Can you work these out from the model? Positions are in its coordinate system, mm. A direction names the side the tool comes from. Coordinates: 2 decimals unless noted, no trailing zeros. Write each loop counter-clockwise with the first axis right and the second up, starting at its lowest first coordinate (ties: lowest second). Pieces come first, ordered by that corner, then holes.
Autodesk Inventor part; units mm, degrees
ref_plane "YZ Plane" through (0, 0, 0) normal (1, 0, 0) x (0, 1, 0)
ref_plane "XZ Plane" through (0, 0, 0) normal (0, 1, 0) x (-1, 0, 0)
ref_plane "XY Plane" through (0, 0, 0) normal (0, 0, 1) x (1, 0, 0)
sketch "Sketch1" plane through (0, 0, 0) normal (0, 0, 1) x (1, 0, 0)
  point P0 (0, 0)
sketch "Sketch2" plane through (0, 0, 0) normal (0, 0, 1) x (1, 0, 0)
  line L0 (0, 0) -> (-34, 0)
  line L1 (-34, 0) -> (-34, 15)
  line L2 (-34, 15) -> (0, 15)
  line L3 (0, 15) -> (0, 0)
  dimension "d0" = 34
  dimension "d1" = 15
extrude "Extrusion1" add sketch "Sketch2" along normal blind 1
sketch "Sketch3" plane through (0, 0, 1) normal (0, 0, 1) x (1, 0, 0)
  line L0 (0, 0) -> (0, 15)
  point P0 (-8, 7.5)
  point P1 (-22, 7.5)
  dimension "d4" = 14
  dimension "d5" = 8
hole "Hole1" at (-22, 7.5, 1) at (-8, 7.5, 1) direction (0, 0, -1) diameter 4.5 end through all
sketch "Sketch4" plane through (0, 0, 1) normal (0, 0, 1) x (1, 0, 0)
  line L0 (-24, 15) -> (-6, 15)
  line L1 (-6, 15) -> (-6, 3)
  line L2 (-6, 3) -> (-24, 3)
  line L3 (-24, 3) -> (-24, 15)
  line L4 (0, 0) -> (0, 15)
  dimension "d13" = 18
  dimension "d14" = 12
  dimension "d15" = 6
extrude "Extrusion2" add sketch "Sketch4" along normal blind 2.8
sketch "Sketch6" plane through (0, 0, 3.8) normal (0, 0, 1) x (1, 0, 0)
  arc A0 (-24, 6.4692) -> (-24, 8.5308) centre (-22, 7.5) ccw
  arc A1 (-6, 8.5308) -> (-6, 6.4692) centre (-8, 7.5) ccw
  point P0 (0, 0)
hole "Hole2" at (-8, 7.5, 3.8) at (-22, 7.5, 3.8) direction (0, 0, -1) diameter 2 end through all
sketch "Sketch5" plane through (0, 0, 3.8) normal (0, 0, 1) x (1, 0, 0)
  line L0 (-34, 15) -> (0, 15)
  line L1 (-18.5, 15) -> (-11.5, 15)
  line L2 (-11.5, 15) -> (-11.5, 3)
  line L3 (-11.5, 3) -> (-18.5, 3)
  line L4 (-18.5, 3) -> (-18.5, 15)
  line L5 (-24, 15) -> (-24, 3)
  line L6 (-6, 3) -> (-6, 15)
  point P0 (0, 0)
  dimension "d18" = 7
  dimension "d19" = 0
  dimension "d20" = 5.5
  dimension "d21" = 5.5
extrude "Extrusion3" add sketch "Sketch5" along normal blind 5.8
sketch "Sketch7" plane through (-34, 15, 0) normal (0, 1, 0) x (1, 0, 0)
  line L0 (0, 0) -> (34, 0)
  line L1 (0, 0) -> (0, -1)
  line L2 (10, -1) -> (0, -1)
  line L3 (10, -1) -> (10, -3.8)
  line L4 (15.5, -3.8) -> (10, -3.8)
  line L5 (15.5, -3.8) -> (15.5, -9.6)
  line L6 (22.5, -9.6) -> (15.5, -9.6)
  line L7 (22.5, -3.8) -> (22.5, -9.6)
  line L8 (28, -3.8) -> (22.5, -3.8)
  line L9 (28, -1) -> (28, -3.8)
  line L10 (34, -1) -> (28, -1)
  line L11 (34, 0) -> (34, -1)
  line L12 (15.5, -3.8) -> (15.5, -9.6)
  line L13 (22.5, -8.35) -> (15.5, -8.35)
  line L14 (15.5, -8.35) -> (15.5, -5)
  line L15 (15.5, -5) -> (22.5, -5)
  line L16 (22.5, -5) -> (22.5, -8.35)
  dimension "d31" = 5
  dimension "d32" = 1.25
extrude "Extrusion4" cut sketch "Sketch7" against normal blind 6 contours L15 L7 L13 L5
sketch "Sketch8" plane through (0, 0, 1) normal (0, 0, 1) x (1, 0, 0)
  point P0 (0, 0)
fillet "Fillet1" radius 1 8 edges at (-34, 0, 0.5) (0, 0, 0.5) (0, 15, 0.5) (-34, 15, 0.5) (-6, 15, 2.4) (-6, 3, 2.4) (-24, 15, 2.4) (-24, 3, 2.4)
move faces "Move1" translate (0, 0, 1) faces at (-18.4872, 1.7718, 0)
properties part number "Z-linear-encoder"
1. If we section it at C-C, the plane y = 7.5: List the corners of the cut face in (x, z) for me.
2. Which directions (+Z, -Z, +X, -X, +Y, -Y) give clear straight access to the entire face, cutting with the end or side of a thin tool? Please do faces 4 (the face through (-18.5, 8, 7)), 5 (the face through (-15, 12, 8.35)), 6 (the face through (-11.5, 8, 7)).
3. If I drill on L1, parallel to X at y = 7.5, z = 2.45; L2, parallel to Z at x = -17.25, y = 12.75; L3, parallel to Y at x = -22, z = 2.6, over which ranges is the centre line in solid material (lowest first)?
4. If we section it at B-B, the plane y = 9.75: List the corners of the cut face in (x, z) for me, plus the area to 4 significant figures.
5. We'd pull the mould along Z, two halves only. Please class faces 1 (the face through (-15, 9, 7)), 2 (the face through (-15, 9, 1)), 3 (the face through (-6.301, 3.285, 2.42)): released by +Z, released by -Z, zero draft, split by the parting line, or undercut.
6. If we section it at A-A, the plane x = -22: List the corners of the cut face in (y, z) for me, plus the area to 3 significant figures.
7. If we section it at D-D, the plane x = -13.5: List the corners of the cut face in (y, z) for me, plus the area to 3 significant figures.
8. I'm going to push flat-ended pins straight in: P1, Ø4.5, axis at x = -22.5, y = 8, coming from the +Z side; P2, Ø1.5, axis at y = 8, z = 7.5, coming from the -X side; P3, Ø2.5, axis at x = -8, y = 7.5, coming from the -Z side; P4, Ø1.7, axis at y = 9.5, z = 5.5, coming from the +X side. Where does each tip first touch, or does it pass through?
Answers:
1. outline: (-24, 1) - (-23, 1) - (-23, 3.8) - (-24, 3.8) - close; (-21, 1) - (-9, 1) - (-9, 3.8) - (-11.5, 3.8) - (-11.5, 9.6) - (-18.5, 9.6) - (-18.5, 3.8) - (-21, 3.8) - close; (-7, 1) - (-6, 1) - (-6, 3.8) - (-7, 3.8) - close
2. face 4: +Z, -X, +Y, -Y
2. face 5: +X, -X, +Y
2. face 6: +Z, +X, +Y, -Y
3. L1: x = -24 to -23, -21 to -9, -7 to -6
3. L2: z = 1 to 5, 8.35 to 9.6
3. L3: y = 3 to 6.5, 8.5 to 15
4. outline: (-24, 1) - (-6, 1) - (-6, 3.8) - (-11.5, 3.8) - (-11.5, 5) - (-18.5, 5) - (-18.5, 3.8) - (-24, 3.8) - close; (-18.5, 8.35) - (-11.5, 8.35) - (-11.5, 9.6) - (-18.5, 9.6) - close
4. area: 67.55 mm2
5. face 1: undercut
5. face 2: released by -Z
5. face 3: zero draft
6. outline: (3, 1) - (6.5, 1) - (6.5, 3.8) - (3, 3.8) - close; (8.5, 1) - (15, 1) - (15, 3.8) - (8.5, 3.8) - close
6. area: 28.0 mm2
7. outline: (3, 1) - (15, 1) - (15, 5) - (9, 5) - (9, 8.35) - (15, 8.35) - (15, 9.6) - (3, 9.6) - close
7. area: 83.1 mm2
8. P1: stops at z = 3.8
8. P2: stops at x = -18.5
8. P3: stops at z = 1
8. P4: stops at x = -11.5
